For this review, use the dimensioned drawing (mm, ordinates from the lowest corner) and the shaded views. A direction names the side the tool comes from. Coordinates: 2 decimals unless noted, no trailing zeros. Order: outer loops, then holes, each group sorted by start corner. A loop starts at its lowest first (then second) coordinate and runs counter-clockwise, first axis right, second up. Notation, with made-up numbers: (37, 45.25) -> (59, 45.25) arc R6 ccw to (59, 56.25) -> close; hole circle Ø8 at (37.25, 81). An arc over 180 degrees is marked (long way). Return JSON: item names as keys, results as strings. Group by question number.
Item 1: Insertion check: pin 1 (2.5 mm diameter, centred on x = 15, y = 55, fed in from -Z). The pin has a flat end and moves straight along its axis. Give the tip position at first contact, or say it passes through.
Item 2: For line 1 along X through (y, z) = (16, 1.2); line 2 along Y through (x, z) = (6, 0.6); line 3 along Y through (x, z) = (12.5, 0.7), list the stretches that pass through material, from the lowest coordinate up.
Item 3: Take a section at D-D (y = 55). Write out the cut boundary in (x, z), then the cut area to 3 significant figures.
Item 4: Draft analysis for pull direction X (two halves, no side actions). For the marked faces 1, 2 and 3, state which applies: +X half, -X half, draft (parallel to the pull), parting line (faces both ways), or undercut.
Item 5: Take a section at C-C (z = 1.75). Write out the cut boundary in (x, y).
Item 6: Machinability: for the marked faces 4 and 5, which of the approach directions +Z, -Z, +X, -X, +Y, -Y give a long, thin tool a straight path to every point of the face, cutting with its end or side? Answer none if there is none.
Item 7: Take a section at A-A (x = 11.25). Write out the cut boundary in (y, z), then the cut area to 3 significant figures.
Item 8: Take a section at B-B (y = 24.5). Write out the cut boundary in (x, z).
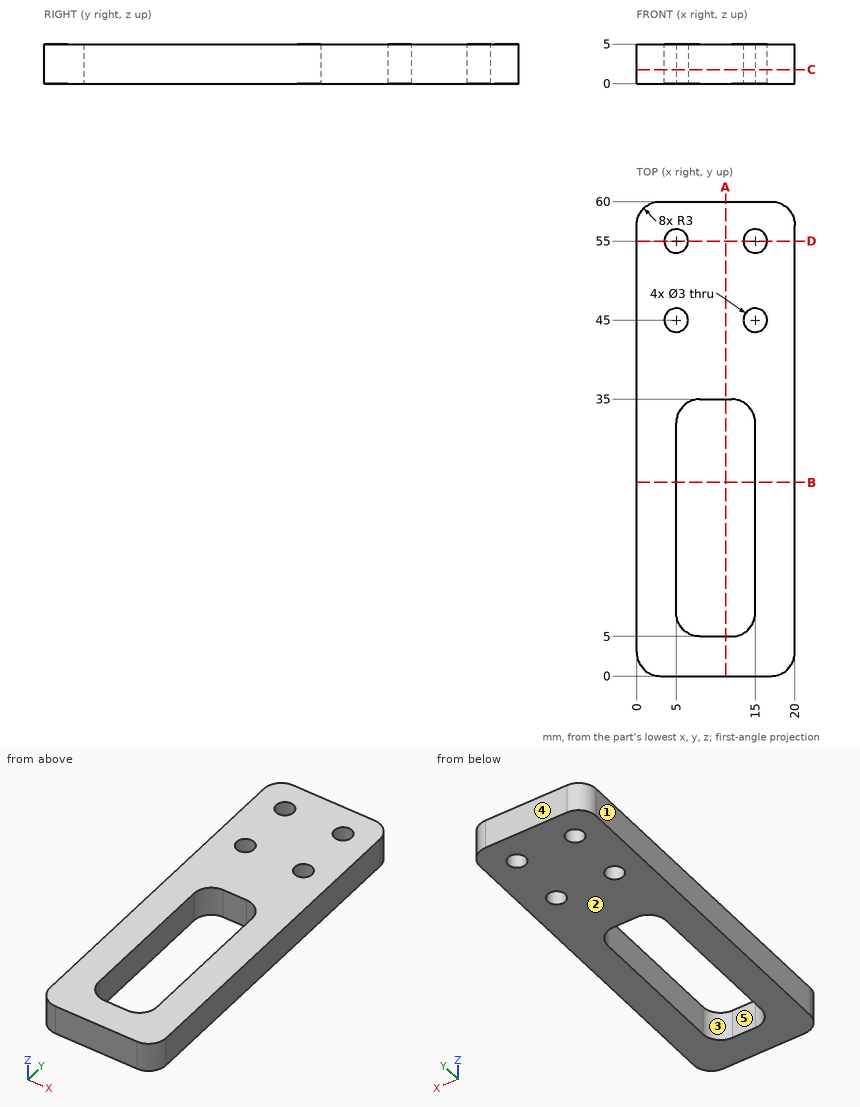
Findings below:
{
 "1": {"pin 1": "passes through"},
 "2": {"line 1": "x = 0 to 5, 15 to 20", "line 2": "y = 0 to 5.76, 34.24 to 43.88, 46.12 to 53.88, 56.12 to 60", "line 3": "y = 0 to 5.04, 34.96 to 60"},
 "3": {"outline": "(0, 0) -> (3.5, 0) -> (3.5, 5) -> (0, 5) -> close; (6.5, 0) -> (13.5, 0) -> (13.5, 5) -> (6.5, 5) -> close; (16.5, 0) -> (20, 0) -> (20, 5) -> (16.5, 5) -> close", "area": "70.0 mm2"},
 "4": {"face 1": "-X half", "face 2": "draft", "face 3": "undercut"},
 "5": {"outline": "(0, 3) arc R3 ccw to (3, 0) -> (17, 0) arc R3 ccw to (20, 3) -> (20, 57) arc R3 ccw to (17, 60) -> (3, 60) arc R3 ccw to (0, 57) -> close; hole circle Ø3 at (5, 45); hole circle Ø3 at (5, 55); hole (5, 8) arc R3 ccw to (8, 5) -> (12, 5) arc R3 ccw to (15, 8) -> (15, 32) arc R3 ccw to (12, 35) -> (8, 35) arc R3 ccw to (5, 32) -> close; hole circle Ø3 at (15, 45); hole circle Ø3 at (15, 55)"},
 "6": {"face 4": "+Z, -Z, +X, -X, +Y", "face 5": "+Z, -Z"},
 "7": {"outline": "(0, 0) -> (5, 0) -> (5, 5) -> (0, 5) -> close; (35, 0) -> (60, 0) -> (60, 5) -> (35, 5) -> close", "area": "150 mm2"},
 "8": {"outline": "(0, 0) -> (5, 0) -> (5, 5) -> (0, 5) -> close; (15, 0) -> (20, 0) -> (20, 5) -> (15, 5) -> close"}
}
